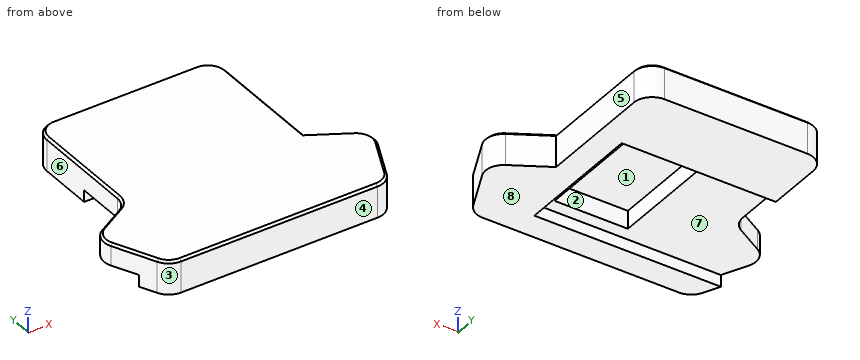
```python
from build123d import *

# Parameters (mm, degrees)
BOSS_EXTRUDE1_DEPTH = 3.2
SKETCH2_W           = 20
SKETCH2_H           = 28
BOSS_EXTRUDE2_DEPTH = 4.9
BOSS_EXTRUDE3_DEPTH = 1
FILLET1_R           = 5
CHAMFER1_SIZE       = 0.6


with BuildPart() as part:
    # Sketch1 → Boss-Extrude1 (new body)
    with BuildSketch(Plane.XY):
        Polygon((-54.5, 42.45), (-12.4, 42.45), (-12.4, 7.25), (-63.3440625, 7.25), (-60, 0), (0, 0), (8.376844495, 18.161180477), (-5.5, 26.172980381), (-5.5, 62.5), (-54.5, 62.5), align=None)
    extrude(amount=BOSS_EXTRUDE1_DEPTH)

    # Sketch2 → Boss-Extrude2 (add)
    with BuildSketch(Plane.XY.offset(3.2)):
        Polygon((-5.5, 26.172980381), (-5.5, 62.5), (-54.5, 62.5), (-54.5, 26.172980381), (-68.376844495, 18.161180477), (-60, 0), (0, 0), (8.376844495, 18.161180477), align=None)
        with Locations((-25.5, 24.85)):
            Rectangle(SKETCH2_W, SKETCH2_H, mode=Mode.SUBTRACT)
    extrude(amount=BOSS_EXTRUDE2_DEPTH)

    # Sketch3 → Boss-Extrude3 (add)
    with BuildSketch(Plane.XY.offset(8.1)):
        Polygon((-68.376844495, 18.161180477), (-60, 0), (0, 0), (8.376844495, 18.161180477), (-5.5, 26.172980381), (-5.5, 62.5), (-54.5, 62.5), (-54.5, 26.172980381), align=None)
    extrude(amount=BOSS_EXTRUDE3_DEPTH)

    # Fillet1
    fillet1_edges = [part.edges().sort_by_distance(p)[0] for p in [
        (-60, 0, 4.55),
        (-54.5, 26.172980381, 6.15),
        (-68.376844495, 18.161180477, 6.15),
        (0, 0, 4.55),
        (8.376844495, 18.161180477, 4.55),
        (-5.5, 62.5, 4.55),
        (-54.5, 62.5, 4.55),
    ]]
    fillet(fillet1_edges, radius=FILLET1_R)

    # Chamfer1
    chamfer1_edges = [part.edges().sort_by_distance(p)[0] for p in [
        (-55.169872981, 26.559731727, 9.1),
        (-5.5, 41.836490191, 9.1),
        (-0.537219377, 23.307717653, 9.1),
        (3.903075742, 8.461952829, 9.1),
        (-60.712780623, 22.586029816, 9.1),
        (-63.903075742, 8.461952829, 9.1),
        (-30, 0, 9.1),
        (-30, 62.5, 9.1),
        (-54.5, 43.279865864, 9.1),
        (-53.035533906, 61.035533906, 9.1),
        (-6.964466094, 61.035533906, 9.1),
        (-66.691006554, 17.625777943, 9.1),
        (-59.495268482, 0.788642997, 9.1),
        (-0.504731518, 0.788642997, 9.1),
        (6.691006554, 17.625777943, 9.1),
    ]]
    chamfer(chamfer1_edges, length=CHAMFER1_SIZE)


solid = part.part
```
The listing builds one solid part. Answer for the finished solid, in the listing's coordinates (mm). Face numbers are marked on the shaded views. A direction names the side the tool comes from. Coordinates: 2 decimals unless noted, no trailing zeros. Write each loop counter-clockwise with the first axis right and the second up, starting at its lowest first coordinate (ties: lowest second). Pieces come first, ordered by that corner, then holes. Notation, with made-up numbers: (68.25, 41) -> (113.25, 41) arc R32 ccw to (113.25, 77) -> close; hole circle Ø6 at (36.5, 89.25). An arc over 180 degrees is marked (long way). Write each question's results on one line, items separated by ' | '. Start each with the question number.
1) Flat-ended cylindrical pins translate along their axes: pin 1 Ø4 at (y, z) = (48, 4.5) entering from +X; pin 2 Ø10.5 at (x, y) = (-41.5, 30.5) entering from -Z; pin 3 Ø4 at (y, z) = (39, 4) entering from -X. Find the tip coordinate at first contact, or state that the pin passes through.
2) For a pull along X with two mould halves and no side action, classify the marked faces 1, 2, 3 and 4 as +X half, -X half, draft (parallel to the pull), parting line (faces both ways), or undercut.
3) A cutting plane is placed at B-B (x = -39). Determine the outline of the cut face in (y, z).
4) A tool of negligible diameter and unlimited length cuts with its end or side. For the marked faces 5, 6, 7 and 8, from which of +Z, -Z, +X, -X, +Y, -Y can it reach the whole face along a straight path? Write none if from no direction.
5) A cutting plane is placed at A-A (z = 5.75). Determine the outline of the cut face in (x, y), then the cut area to 3 significant figures.
6) A cutting plane is placed at D-D (z = 1.75). Determine the outline of the cut face in (x, y).
7) Straight lines are drawn through the part: probe 1 along Y at (x, z) = (-27, 7.25); probe 2 along X at (y, z) = (16, 5.25); probe 3 along X at (y, z) = (30, 2.5). For each, find the intervals that lie inside material, in ascending order.
8) A cutting plane is placed at C-C (y = 38). Determine the outline of the cut face in (x, z).
Values follow:
1) pin 1: x = -5.5 | pin 2: z = 3.2 | pin 3: x = -54.5
2) face 1: undercut | face 2: undercut | face 3: -X half | face 4: draft
3) outline: (0, 0) -> (7.25, 0) -> (7.25, 3.2) -> (42.45, 3.2) -> (42.45, 0) -> (62.5, 0) -> (62.5, 8.5) -> (61.9, 9.1) -> (0.6, 9.1) -> (0, 8.5) -> close
4) face 5: +Z, -Z, +X, +Y | face 6: +Z, -Z, -X, +Y | face 7: -Z, -X | face 8: -Z, +X, -X, +Y, -Y
5) outline: (-66.47, 14.02) -> (-61.34, 2.91) arc R5 ccw to (-56.8, 0) -> (-3.2, 0) arc R5 ccw to (1.34, 2.91) -> (6.47, 14.02) arc R5 ccw to (4.43, 20.44) -> (-5.5, 26.17) -> (-5.5, 57.5) arc R5 ccw to (-10.5, 62.5) -> (-49.5, 62.5) arc R5 ccw to (-54.5, 57.5) -> (-54.5, 29.06) arc R5 cw to (-57, 24.73) -> (-64.43, 20.44) arc R5 ccw to start; hole (-35.5, 10.85) -> (-15.5, 10.85) -> (-15.5, 38.85) -> (-35.5, 38.85) -> close | area: 2,940 mm²
6) outline: (-63.34, 7.25) -> (-61.34, 2.91) arc R5 ccw to (-56.8, 0) -> (-3.2, 0) arc R5 ccw to (1.34, 2.91) -> (6.47, 14.02) arc R5 ccw to (4.43, 20.44) -> (-5.5, 26.17) -> (-5.5, 57.5) arc R5 ccw to (-10.5, 62.5) -> (-49.5, 62.5) arc R5 ccw to (-54.5, 57.5) -> (-54.5, 42.45) -> (-12.4, 42.45) -> (-12.4, 7.25) -> close
7) probe 1: 0 to 10.85, 38.85 to 62.5 | probe 2: -66.92 to -35.5, -15.5 to 6.92 | probe 3: -12.4 to -5.5
8) outline: (-54.5, 3.2) -> (-35.5, 3.2) -> (-35.5, 8.1) -> (-15.5, 8.1) -> (-15.5, 3.2) -> (-12.4, 3.2) -> (-12.4, 0) -> (-5.5, 0) -> (-5.5, 8.5) -> (-6.1, 9.1) -> (-53.9, 9.1) -> (-54.5, 8.5) -> close
